```python
from build123d import *

# Parameters (mm, degrees)
F0_W     = 78.15
F0_H     = 43.1
F1_DEPTH = 19.23
F2_W     = 65.97
F2_H     = 36.84
F3_DEPTH = 35
F4_R     = 1.5
F5_DEPTH = 100000
F8_DEPTH = 2
F9_DEPTH = 2


with BuildPart() as f1:
    # F0 (on Front) → F1 (new body)
    with BuildSketch(Plane.XZ):
        Rectangle(F0_W, F0_H)
    extrude(amount=F1_DEPTH)

    # F2 (on face) → F3 (cut)
    with BuildSketch(Plane.XZ.offset(19.23)):
        Rectangle(F2_W, F2_H)
    extrude(amount=-F3_DEPTH, mode=Mode.SUBTRACT)

    # F4 (on face) → F5 (cut)
    with BuildSketch(Plane.YZ.offset(39.075)):
        with Locations((-9.615, 11.38)):
            Circle(F4_R)
        with Locations((-9.615, -11.38)):
            Circle(F4_R)
    extrude(amount=-F5_DEPTH, mode=Mode.SUBTRACT)

    # F7 (on face) → F8 (cut)
    with BuildSketch(Plane(origin=(32.985, 0, 0), x_dir=(0, -1, 0), z_dir=(-1, 0, 0))):
        Polygon((12.365, 9.792287), (12.365, 12.967713), (9.615, 14.555426), (6.865, 12.967713), (6.865, 9.792287), (9.615, 8.204574), align=None)
        Polygon((6.865, -12.967713), (9.615, -14.555426), (12.365, -12.967713), (12.365, -9.792287), (9.615, -8.204574), (6.865, -9.792287), align=None)
    extrude(amount=-F8_DEPTH, mode=Mode.SUBTRACT)

    # F6 (on face) → F9 (cut)
    with BuildSketch(Plane.YZ.offset(-32.985)):
        Polygon((-6.865, 9.792287), (-6.865, 12.967713), (-9.615, 14.555426), (-12.365, 12.967713), (-12.365, 9.792287), (-9.615, 8.204574), align=None)
        Polygon((-12.365, -12.967713), (-9.615, -14.555426), (-6.865, -12.967713), (-6.865, -9.792287), (-9.615, -8.204574), (-12.365, -9.792287), align=None)
    extrude(amount=-F9_DEPTH, mode=Mode.SUBTRACT)


solid = f1.part
```
Build history of the part. All positions in model axes, mm. A direction names the side the tool comes from. Round coordinates to 2 decimals unless told otherwise and drop trailing zeros. Order: outer loops, then holes, each group sorted by start corner. A loop starts at its lowest first (then second) coordinate and runs counter-clockwise, first axis right, second up. Notation, with made-up numbers: (28.5, 33.25) -> (49.5, 33.25) arc R28 ccw to (49.5, 61.25) -> close; hole circle Ø4 at (65, 37.5). An arc over 180 degrees is marked (long way). Answer in a Markdown table with one row per item.
1) Band-saw the part on A-A on z = -16. Give the cut face in (x, y) (3 decimals).
Values:
| item | result |
|---|---|
| outline | (-39.075, -19.23) -> (-32.985, -19.23) -> (-32.985, 0) -> (-39.075, 0) -> close; (32.985, -19.23) -> (39.075, -19.23) -> (39.075, 0) -> (32.985, 0) -> close |
2) Band-saw the part on B-B on x = 3. Give the cut face in (y, z).
Values:
| item | result |
|---|---|
| outline | (-19.23, -21.55) -> (0, -21.55) -> (0, -18.42) -> (-19.23, -18.42) -> close; (-19.23, 18.42) -> (0, 18.42) -> (0, 21.55) -> (-19.23, 21.55) -> close |
3) Band-saw the part on C-C on z = 11.38. Give the cut face in (x, y) (3 decimals), and give its area (3 significant figures).
Values:
| item | result |
|---|---|
| outline | (-39.075, -19.23) -> (-32.985, -19.23) -> (-32.985, -12.365) -> (-34.985, -12.365) -> (-34.985, -11.115) -> (-39.075, -11.115) -> close; (-39.075, -8.115) -> (-34.985, -8.115) -> (-34.985, -6.865) -> (-32.985, -6.865) -> (-32.985, 0) -> (-39.075, 0) -> close; (32.985, -19.23) -> (39.075, -19.23) -> (39.075, -11.115) -> (34.985, -11.115) -> (34.985, -12.365) -> (32.985, -12.365) -> close; (32.985, -6.865) -> (34.985, -6.865) -> (34.985, -8.115) -> (39.075, -8.115) -> (39.075, 0) -> (32.985, 0) -> close |
| area | 188 mm2 |
4) Which spindle directions (+Z, -Z, +X, -X, +Y, -Y) get a long thin tool onto all of the face, cutting with end or side? Do faces 4 (the cylindrical face through (-37.001, -11.114, -11.314)), 5 (the flat face through (33.97, -11.01, 13.75)), 6 (the flat face through (-32.985, -10, 0)). Say none if no direction does.
Values:
| item | result |
|---|---|
| face 4 | +X, -X |
| face 5 | none |
| face 6 | +Y, -Y |
5) Pin check, flat tip, straight feed: P1, Ø6, axis at x = -28.5, z = -14, coming from the +Y side. Stop position of the tip, or through.
Values:
| item | result |
|---|---|
| P1 | through |
6) Mould opens along X. For faces 1 (the flat face through (-1, -19.23, -19)), 2 (the flat face through (0, -10, -18.42)), 3 (the flat face through (33.971, -10.971, -13.773)) say: released by +X, released by -X, zero draft, split by the parting line, or undercut.
Values:
| item | result |
|---|---|
| face 1 | zero draft |
| face 2 | undercut |
| face 3 | undercut |
7) Band-saw the part on D-D on y = -16. Give the cut face in (x, z) (3 decimals).
Values:
| item | result |
|---|---|
| outline | (-39.075, -21.55) -> (39.075, -21.55) -> (39.075, 21.55) -> (-39.075, 21.55) -> close; hole (-32.985, -18.42) -> (32.985, -18.42) -> (32.985, 18.42) -> (-32.985, 18.42) -> close |
8) Wall check: L1, parallel to Z at x = 17.5, y = -15.75; L2, parallel to X at y = -13.5, z = -12 (3 decimals). Give the ranges that are in metal, low to high.
Values:
| item | result |
|---|---|
| L1 | -21.55 to -18.42, 18.42 to 21.55 |
| L2 | -39.075 to -32.985, 32.985 to 39.075 |
